Design review of the part built by this model. Coordinates are the model's own, in mm. Coordinates: 2 decimals unless noted, no trailing zeros. Order: outer loops, then holes, each group sorted by start corner. A loop starts at its lowest first (then second) coordinate and runs counter-clockwise, first axis right, second up. Notation, with made-up numbers: M 64.25,85 L 89.25,85 A26 ccw 89.25,107 Z; hole C -4,86.5 d1. An arc over 180 degrees is marked long. Answer as a JSON object with one key per item and string values.
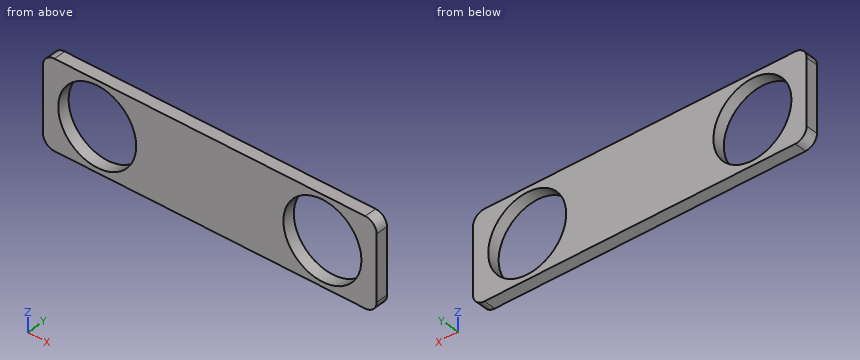
from build123d import *

# Parameters (mm, degrees)
SKETCH1_W           = 87.682
SKETCH1_H           = 23
SKETCH1_R           = 10.25
BOSS_EXTRUDE1_DEPTH = 3.2
FILLET1_R           = 3


with BuildPart() as part:
    # Sketch1 → Boss-Extrude1 (new body)
    with BuildSketch(Plane(origin=(0, 0, 0), x_dir=(1, 0, 0), z_dir=(0, 1, 0))):
        Rectangle(SKETCH1_W, SKETCH1_H)
        with Locations(Location((29.591, 0, 0), (0, 0, 270))):
            Circle(SKETCH1_R, mode=Mode.SUBTRACT)
        with Locations(Location((-29.591, 0, 0), (0, 0, 270))):
            Circle(SKETCH1_R, mode=Mode.SUBTRACT)
    extrude(amount=BOSS_EXTRUDE1_DEPTH)

    # Fillet1
    fillet1_edges = [part.edges().sort_by_distance(p)[0] for p in [
        (43.841, 1.6, -11.5),
        (43.841, 1.6, 11.5),
        (-43.841, 1.6, 11.5),
        (-43.841, 1.6, -11.5),
    ]]
    fillet(fillet1_edges, radius=FILLET1_R)


solid = part.part
1) To check wall thickness, follow L1, parallel to X at y = 2.3, z = 0; L2, parallel to X at y = 0.7, z = -6; L3, parallel to Z at x = -24.5, y = 0.5. State the ranges of each line that lie inside material, in increasing order.
Taken from the geometry:
{"L1": "x = -43.84 to -39.84, -19.34 to 19.34, 39.84 to 43.84", "L2": "x = -43.84 to -37.9, -21.28 to 21.28, 37.9 to 43.84", "L3": "z = -11.5 to -8.9, 8.9 to 11.5"}
2) Add section C-C (y = 0.9). State the section outline as (x, z) points, and give its area (3 significant figures).
Taken from the geometry:
{"outline": "M -43.84,-8.5 A3 ccw -40.84,-11.5 L 40.84,-11.5 A3 ccw 43.84,-8.5 L 43.84,8.5 A3 ccw 40.84,11.5 L -40.84,11.5 A3 ccw -43.84,8.5 Z; hole C -29.59,0 d20.5; hole C 29.59,0 d20.5", "area": "1,350 mm2"}
3) Add section A-A (z = 0). State the section outline as (x, y) points, and give its area (3 significant figures).
Taken from the geometry:
{"outline": "M -43.84,0 L -39.84,0 L -39.84,3.2 L -43.84,3.2 Z; M -19.34,0 L 19.34,0 L 19.34,3.2 L -19.34,3.2 Z; M 39.84,0 L 43.84,0 L 43.84,3.2 L 39.84,3.2 Z", "area": "149 mm2"}
4) Add section D-D (z = 3.25). State the section outline as (x, y) points.
Taken from the geometry:
{"outline": "M -43.84,0 L -39.31,0 L -39.31,3.2 L -43.84,3.2 Z; M -19.87,0 L 19.87,0 L 19.87,3.2 L -19.87,3.2 Z; M 39.31,0 L 43.84,0 L 43.84,3.2 L 39.31,3.2 Z"}
5) Add section B-B (x = 35.5). State the section outline as (y, z) points.
Taken from the geometry:
{"outline": "M 0,-11.5 L 3.2,-11.5 L 3.2,-8.38 L 0,-8.38 Z; M 0,8.38 L 3.2,8.38 L 3.2,11.5 L 0,11.5 Z"}
